Build history of the part. All positions in model axes, mm. Face numbers are marked on the shaded views. A direction names the side the tool comes from. Coordinates: 2 decimals unless noted, no trailing zeros. Order: outer loops, then holes, each group sorted by start corner. A loop starts at its lowest first (then second) coordinate and runs counter-clockwise, first axis right, second up. Notation, with made-up numbers: (11, 9) - (64, 9) arc R18 ccw to (64, 34) - close; hole circle Ø9 at (-2, 3.5). An arc over 180 degrees is marked (long way). One line per item, written item: value.
from build123d import *

# Parameters (mm, degrees)
SKETCH1_W           = 46
SKETCH1_H           = 46
BOSS_EXTRUDE1_DEPTH = 11
SKETCH3_R           = 19
BOSS_EXTRUDE3_DEPTH = 4.5
CUT_EXTRUDE1_START  = -3
SKETCH4_R           = 16
CUT_EXTRUDE1_DEPTH  = 4
SKETCH5_R           = 12.5
CUT_EXTRUDE2_DEPTH  = 29
SKETCH6_R           = 8
BOSS_EXTRUDE4_DEPTH = 12
SKETCH6_3_R         = 6
BOSS_EXTRUDE5_DEPTH = 22
FILLET1_R           = 3


with BuildPart() as part:
    # Sketch1 → Boss-Extrude1 (new body, symmetric)
    with BuildSketch(Plane(origin=(0, 0, 0), x_dir=(1, 0, 0), z_dir=(0, 1, 0))):
        Rectangle(SKETCH1_W, SKETCH1_H)
    extrude(amount=BOSS_EXTRUDE1_DEPTH, both=True)

    # Sketch3 → Boss-Extrude3 (add)
    with BuildSketch(Plane(origin=(0, 11, 0), x_dir=(1, 0, 0), z_dir=(0, 1, 0))):
        Circle(SKETCH3_R)
    boss_extrude3 = extrude(amount=BOSS_EXTRUDE3_DEPTH)

    # Mirror1: Boss-Extrude3 across plane
    add(boss_extrude3.mirror(Plane.ZX))

    # Sketch4 → Cut-Extrude1 (cut)
    with BuildSketch(Plane(origin=(0, 15.5, 0), x_dir=(1, 0, 0), z_dir=(0, 1, 0)).offset(CUT_EXTRUDE1_START)):
        Circle(SKETCH4_R)
    cut_extrude1 = extrude(amount=CUT_EXTRUDE1_DEPTH, mode=Mode.SUBTRACT)

    # Mirror2: Cut-Extrude1 across plane
    add(cut_extrude1.mirror(Plane.ZX), mode=Mode.SUBTRACT)

    # Sketch5 → Cut-Extrude2 (cut, through all)
    with BuildSketch(Plane(origin=(0, 12.5, 0), x_dir=(1, 0, 0), z_dir=(0, 1, 0))):
        Circle(SKETCH5_R)
    extrude(amount=-CUT_EXTRUDE2_DEPTH, mode=Mode.SUBTRACT)

    # Sketch6 → Boss-Extrude4 (add)
    with BuildSketch(Plane(origin=(23, 0, 0), x_dir=(0, 0, -1), z_dir=(1, 0, 0))):
        Circle(SKETCH6_R)
    boss_extrude4 = extrude(amount=BOSS_EXTRUDE4_DEPTH)

    # Sketch6<3> → Boss-Extrude5 (add)
    with BuildSketch(Plane(origin=(23, 0, 0), x_dir=(0, 0, -1), z_dir=(1, 0, 0))):
        Circle(SKETCH6_3_R)
    boss_extrude5 = extrude(amount=BOSS_EXTRUDE5_DEPTH)

    # Mirror3: Boss-Extrude4, Boss-Extrude5 across plane
    add(boss_extrude4.mirror(Plane(origin=(0, 0, 0), x_dir=(0, 0, 1), z_dir=(1, 0, 0))))
    add(boss_extrude5.mirror(Plane(origin=(0, 0, 0), x_dir=(0, 0, 1), z_dir=(1, 0, 0))))

    # Fillet1
    fillet1_edges = [part.edges().sort_by_distance(p)[0] for p in [
        (-19, 11, 0),
        (-19, -11, 0),
    ]]
    fillet(fillet1_edges, radius=FILLET1_R)


solid = part.part
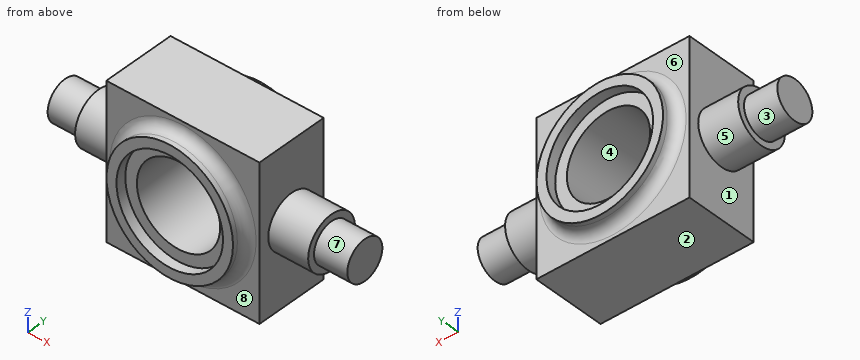
1. Probe line 1 along Z through (x, y) = (0, 14.75); line 2 along Z through (x, y) = (0, 7.5). List the from-to ranges inside material, lowest first.
Values found:
line 1: z = -19 to -16, 16 to 19
line 2: z = -23 to -12.5, 12.5 to 23
2. 3-axis set-ups, long thin cutter, end or side, ignore diameter. For the marked faces 5, 6, 7 and 8: which of +Z, -Z, +X, -X, +Y, -Y reach the whole face in a straight line?
Values found:
face 5: -X
face 6: +Y
face 7: +X
face 8: -Y
3. Flat gauge pins, fed straight in: P1, Ø10, axis at y = -2.5, z = -13, coming from the +X side; P2, Ø4, axis at x = -24, z = -3.5, coming from the -Y side; P3, Ø4, axis at x = 13, z = 2.5, coming from the +Y side; P4, Ø8, axis at y = -5.5, z = 3, coming from the -X side. Where does each tip first touch, or does it go through?
Values found:
P1: stops at x = 23
P2: stops at y = -11
P3: stops at y = 12.5
P4: stops at x = -45
4. Band-saw the part on D-D, the plane y = -9. Give the cut face in (x, z).
Values found:
outline: (-23, -23) - (23, -23) - (23, 23) - (-23, 23) - close; hole circle Ø25 at (0, 0)
5. Band-saw the part on C-C, the plane x = 39. Give the cut face in (y, z).
Values found:
outline: circle Ø12 at (0, 0)
6. Band-saw the part on A-A, the plane y = 0. Give the cut face in (x, z), and give its area (3 significant figures).
Values found:
outline: (-45, -6) - (-35, -6) - (-35, -8) - (-23, -8) - (-23, -23) - (23, -23) - (23, -8) - (35, -8) - (35, -6) - (45, -6) - (45, 6) - (35, 6) - (35, 8) - (23, 8) - (23, 23) - (-23, 23) - (-23, 8) - (-35, 8) - (-35, 6) - (-45, 6) - close; hole circle Ø25 at (0, 0)
area: 2,250 mm2
7. Two-plate mould, pull along Z, no slides. Class the marked faces 1, 2, 3 and 4: pulls with the +Z half, pulls with the -Z half, needs draft (parallel to the pull), parting line crosses it, or undercut.
Values found:
face 1: needs draft
face 2: pulls with the -Z half
face 3: parting line crosses it
face 4: undercut
8. Band-saw the part on B-B, the plane x = 0. Give the cut face in (y, z), and give its area (3 significant figures).
Values found:
outline: (-15.5, -19) - (-14, -19) arc R3 cw to (-11, -22) - (-11, -23) - (11, -23) - (11, -22) arc R3 cw to (14, -19) - (15.5, -19) - (15.5, -16) - (12.5, -16) - (12.5, -12.5) - (-12.5, -12.5) - (-12.5, -16) - (-15.5, -16) - close; (-15.5, 16) - (-12.5, 16) - (-12.5, 12.5) - (12.5, 12.5) - (12.5, 16) - (15.5, 16) - (15.5, 19) - (14, 19) arc R3 cw to (11, 22) - (11, 23) - (-11, 23) - (-11, 22) arc R3 cw to (-14, 19) - (-15.5, 19) - close
area: 545 mm2
